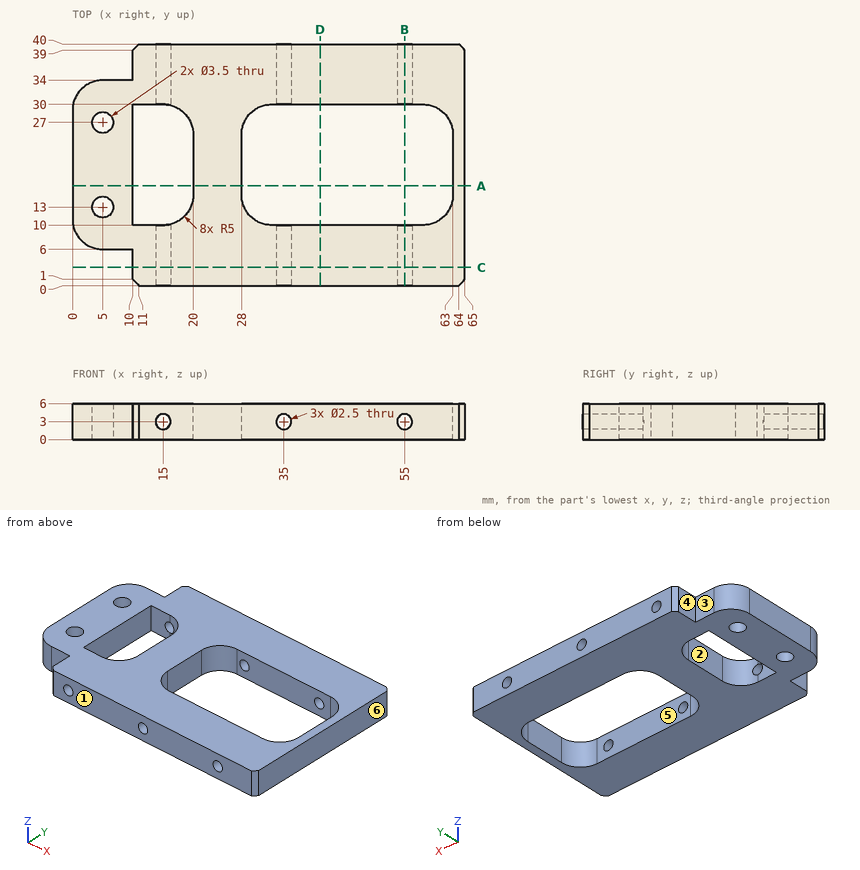
Source: three-view drawing plus pictorial views. Frame: mm from the lowest corner of the part. A direction names the side the tool comes from. Coordinates: 2 decimals unless noted, no trailing zeros. Loops run counter-clockwise (first coordinate to the right, second up) from the corner with the lowest first, then second, coordinate; pieces in that order, holes last. Notation, with made-up numbers: (30.5, 77) - (38.5, 77) arc R14 ccw to (38.5, 103) - close; hole circle Ø3 at (-2, 11.5). An arc over 180 degrees is marked (long way). One line per item, written item: value. Start each with the question number.
1. Section B-B (x = 55). Return the cut outline in (y, z).
2. Set-up query: the marked faces 1, 2 and 3. Return all of +Z, -Z, +X, -X, +Y, -Y with unobstructed straight access to the full face (end or side cutting, diameter ignored); none if empty.
3. Contact query for flat-ended pins moving along their axis: P1, Ø2, axis at y = 28.5, z = 4.5, coming from the -X side; P2, Ø2.5, axis at x = 6.5, z = 3, coming from the -Y side; P3, Ø2.5, axis at x = 8, z = 2, coming from the +Y side. Output: stop coordinate, or through.
4. Section D-D (x = 41). Return the cut outline in (y, z), and give its area (3 significant figures).
5. Mould query, pull axis X, two halves, no side actions, for the marked faces 4, 5 and 6. Classes: pulls with the +X half, pulls with the -X half, needs draft (parallel to the pull), parting line crosses it, or undercut.
6. Section C-C (y = 3). Return the cut outline in (x, z), and give its area (3 significant figures).
7. Section A-A (y = 16.5). Return the cut outline in (x, z), and give its area (3 significant figures).
8. Ray query, L1, parallel to X at y = 16, z = 3; L2, parallel to Y at x = 5, z = 4.55; L3, parallel to X at y = 31, z = 2.25. Return the intervals inside material, ascending.
Verdict:
1. outline: (0, 0) - (10, 0) - (10, 1.75) - (0, 1.75) - close; (0, 4.25) - (10, 4.25) - (10, 6) - (0, 6) - close; (30, 0) - (40, 0) - (40, 1.75) - (30, 1.75) - close; (30, 4.25) - (40, 4.25) - (40, 6) - (30, 6) - close
2. face 1: +Z, -Z, +X, -X, -Y
2. face 2: +Z, -Z
2. face 3: +Z, -Z, -X, +Y
3. P1: stops at x = 0
3. P2: stops at y = 6
3. P3: stops at y = 34
4. outline: (0, 0) - (10, 0) - (10, 6) - (0, 6) - close; (30, 0) - (40, 0) - (40, 6) - (30, 6) - close
4. area: 120 mm2
5. face 4: pulls with the -X half
5. face 5: undercut
5. face 6: pulls with the +X half
6. outline: (10, 0) - (65, 0) - (65, 6) - (10, 6) - close; hole circle Ø2.5 at (15, 3); hole circle Ø2.5 at (35, 3); hole circle Ø2.5 at (55, 3)
6. area: 315 mm2
7. outline: (0, 0) - (10, 0) - (10, 6) - (0, 6) - close; (20, 0) - (28, 0) - (28, 6) - (20, 6) - close; (63, 0) - (65, 0) - (65, 6) - (63, 6) - close
7. area: 120 mm2
8. L1: x = 0 to 10, 20 to 28, 63 to 65
8. L2: y = 6 to 11.25, 14.75 to 25.25, 28.75 to 34
8. L3: x = 0.42 to 14, 16 to 34, 36 to 54, 56 to 65
